Verification items for the finished model (mm, model axes). Face numbers are marked on the shaded views. Give positions to 0.01 mm unless a question says otherwise; leave off trailing zeros. Write each loop counter-clockwise with the first axis right and the second up, starting at its lowest first coordinate (ties: lowest second). Pieces come first, ordered by that corner, then holes. Notation, with made-up numbers: (-19, 21.25) - (33, 21.25) arc R22 ccw to (33, 29.25) - close; hole circle Ø10 at (18, 51.5). An arc over 180 degrees is marked (long way). Answer as a JSON object with one key per item and string values. Group by question number.
Item 1: Draft check along Z on the marked faces 1 and 2. Enter one of: +Z half, -Z half, draft (parallel to the pull), parting line (faces both ways), or undercut.
Item 2: Sectioned sample at B-B, the plane x = 936.5. Record the boundary of the cut face in (y, z), and give its area (4 significant figures).
Item 3: Sectioned sample at C-C, the plane y = -162. Count the separate pieces of the cut face and the enclosed holes in it, and give its area (3 significant figures).
Item 4: Scan lines: line 1 along X through (y, z) = (-86.5, 270.5); line 2 along Z through (x, y) = (179.5, -322). Record each from-to range of solid material in increasing order. Write a range as [from, to].
Item 5: Sectioned sample at A-A, the plane z = 497. Record the boundary of the cut face in (x, y), and give its area (3 significant figures).
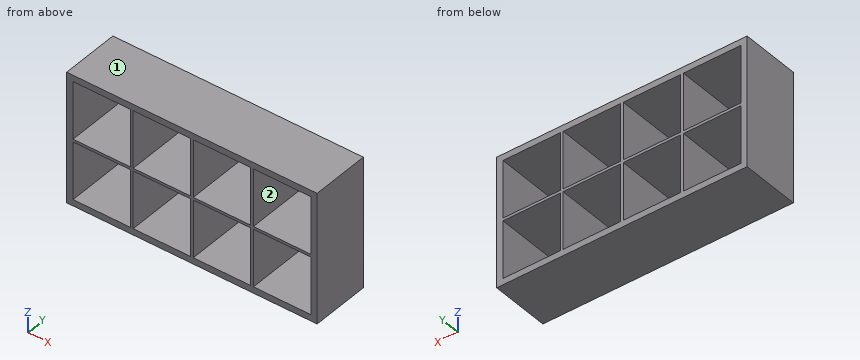
```python
from build123d import *

# Parameters (mm, degrees)
F0_W     = 37
F0_H     = 382.5875
F1_DEPTH = 345
F2_W     = 345
F2_H     = 37
F3_DEPTH = 698
F7_W     = 345
F7_H     = 8
F8_DEPTH = 698
F4_W     = 16
F4_H     = 345
F4_W_2   = 8
F5_DEPTH = 337.5875


with BuildPart() as f1:
    # F0 (on Front) → F1 (new body)
    with BuildSketch(Plane.XZ):
        with Locations((-20.093406, 89.323638)):
            Rectangle(F0_W, F0_H)
    extrude(amount=F1_DEPTH)

    # F2 (on face) → F3 (join)
    with BuildSketch(Plane.YZ.offset(-1.593406)):
        with Locations((-172.5, -83.470112)):
            Rectangle(F2_W, F2_H)
    extrude(amount=F3_DEPTH)

    # F7 (on face) → F8 (join)
    with BuildSketch(Plane.YZ.offset(-1.593406)):
        with Locations((-172.5, 276.617388)):
            Rectangle(F7_W, F7_H)
    extrude(amount=F8_DEPTH)

    # F4 (on face) → F5 (join, through all)
    with BuildSketch(Plane.XY.offset(-64.970112)):
        with Locations((343.406594, -172.5)):
            Rectangle(F4_W, F4_H)
        with Locations((692.406594, -172.5)):
            Rectangle(F4_W_2, F4_H)
    extrude(amount=F5_DEPTH)

    # F9: F1 across face


with BuildPart() as f1_1:
    add(f1.part)
    add(f1.part.mirror(Plane(origin=(328.906594, -172.5, 280.617388), x_dir=(1, 0, 0), z_dir=(0, 0, 1))))

    # F6: F1 across face


with BuildPart() as f1_2:
    add(f1_1.part)
    add(f1_1.part.mirror(Plane(origin=(696.406594, -172.5, 280.617388), x_dir=(0, 1, 0), z_dir=(1, 0, 0))))


solid = f1_2.part
```
Geometry check:
{
 "1": {"face 1": "+Z half", "face 2": "undercut"},
 "2": {"outline": "(-345, -101.97) - (0, -101.97) - (0, -64.97) - (-345, -64.97) - close; (-345, 272.62) - (0, 272.62) - (0, 288.62) - (-345, 288.62) - close; (-345, 626.2) - (0, 626.2) - (0, 663.2) - (-345, 663.2) - close", "area": "31,050 mm^2"},
 "3": {"separate pieces": "1", "enclosed holes": "8", "area": "215,000 mm^2"},
 "4": {"line 1": "[-38.59, -1.59], [335.41, 351.41], [688.41, 704.41], [1041.41, 1057.41], [1394.41, 1431.41]", "line 2": "[-101.97, -64.97], [272.62, 288.62], [626.2, 663.2]"},
 "5": {"outline": "(-38.59, -345) - (-1.59, -345) - (-1.59, 0) - (-38.59, 0) - close; (335.41, -345) - (351.41, -345) - (351.41, 0) - (335.41, 0) - close; (688.41, -345) - (704.41, -345) - (704.41, 0) - (688.41, 0) - close; (1041.41, -345) - (1057.41, -345) - (1057.41, 0) - (1041.41, 0) - close; (1394.41, -345) - (1431.41, -345) - (1431.41, 0) - (1394.41, 0) - close", "area": "42,100 mm^2"}
}
